Verification items for the finished model (mm, model axes). Face numbers are marked on the shaded views. A direction names the side the tool comes from. Give positions to 0.01 mm unless a question says otherwise; leave off trailing zeros. Order: outer loops, then holes, each group sorted by start corner. A loop starts at its lowest first (then second) coordinate and runs counter-clockwise, first axis right, second up. Notation, with made-up numbers: (62.25, 75.25) - (118.25, 75.25) arc R26 ccw to (118.25, 108.25) - close; hole circle Ø7 at (24, -5.5). An arc over 180 degrees is marked (long way). Answer as a JSON object with one key per item and string values.
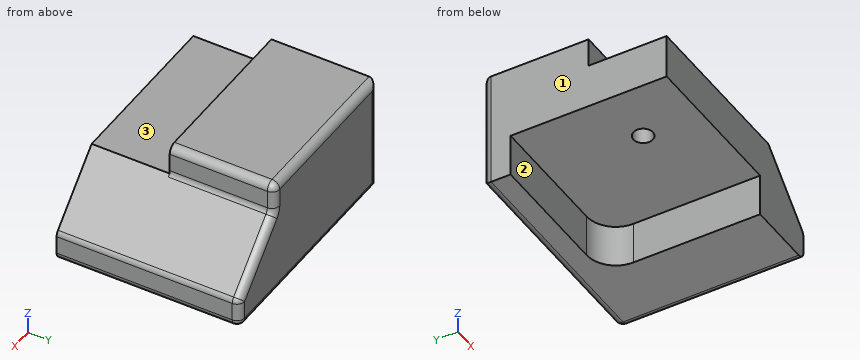
```python
from build123d import *

# Parameters (mm, degrees)
SKETCH2_W           = 14.859
SKETCH2_H           = 11.938
BOSS_EXTRUDE1_DEPTH = 7.62
CUT_EXTRUDE2_DEPTH  = 2.794
CUT_EXTRUDE3_DEPTH  = 1.905
CUT_EXTRUDE4_DEPTH  = 12.938
FILLET1_R           = 0.508
SKETCH7_R           = 0.635
CUT_EXTRUDE13_DEPTH = 1.905


with BuildPart() as part:
    # Sketch2 → Boss-Extrude1 (new body)
    with BuildSketch(Plane.XY):
        with Locations((7.4295, 5.969)):
            Rectangle(SKETCH2_W, SKETCH2_H)
    extrude(amount=BOSS_EXTRUDE1_DEPTH)

    # Sketch4 → Cut-Extrude2 (cut)
    with BuildSketch(Plane(origin=(0, 0, 0), x_dir=(-1, 0, 0), z_dir=(0, 0, -1))):
        with BuildLine():
            Line((0, 0), (-10.16, 0))
            Line((-10.16, 0), (-10.16, 8.255))
            ThreePointArc((-10.16, 8.255), (-9.602038418, 9.602038418), (-8.255, 10.16))
            Line((-8.255, 10.16), (0, 10.16))
            Line((0, 10.16), (0, 0))
        make_face()
    extrude(amount=-CUT_EXTRUDE2_DEPTH, mode=Mode.SUBTRACT)

    # Sketch5 → Cut-Extrude3 (cut)
    with BuildSketch(Plane.XY.offset(7.62)):
        Polygon((14.859, 11.938), (11.049, 11.938), (11.049, 5.08), (0, 5.08), (0, 0), (14.859, 0), align=None)
    extrude(amount=-CUT_EXTRUDE3_DEPTH, mode=Mode.SUBTRACT)

    # Sketch6 → Cut-Extrude4 (cut, through all)
    with BuildSketch(Plane(origin=(0, 11.938, 0), x_dir=(1, 0, 0), z_dir=(0, 1, 0))):
        Polygon((14.859, -1.905), (11.049, -5.715), (14.859, -5.715), align=None)
    extrude(amount=-CUT_EXTRUDE4_DEPTH, mode=Mode.SUBTRACT)

    # Fillet1
    fillet1_edges = [part.edges().sort_by_distance(p)[0] for p in [
        (5.5245, 11.938, 7.62),
        (11.049, 11.938, 6.6675),
        (11.049, 8.509, 5.715),
        (11.049, 8.509, 7.62),
        (7.4295, 11.938, 0),
        (14.859, 11.938, 0.9525),
        (14.859, 5.969, 0),
        (12.954, 11.938, 3.81),
        (14.859, 5.969, 1.905),
        (0, 11.938, 3.81),
    ]]
    fillet(fillet1_edges, radius=FILLET1_R)

    # Sketch7 → Cut-Extrude13 (cut)
    with BuildSketch(Plane(origin=(0, 0, 2.794), x_dir=(-1, 0, 0), z_dir=(0, 0, -1))):
        with Locations((-3.81, 3.81)):
            Circle(SKETCH7_R)
    extrude(amount=-CUT_EXTRUDE13_DEPTH, mode=Mode.SUBTRACT)


solid = part.part
```
(1) Access from +Z, -Z, +X, -X, +Y, -Y to the whole of each face (thin tool, end or side, straight path). Record for the marked faces 1, 2 and 3.
Computed values:
{"face 1": "+Z, -Z, -X, +Y, -Y", "face 2": "-Z, -X, -Y", "face 3": "+Z, +X, -X, -Y"}
(2) Section check D-D (y = 0.5). Record the cut outline in (x, z) (3 decimals), then the cut area to 3 significant figures.
Computed values:
{"outline": "(0, 2.794) - (10.16, 2.794) - (10.16, 0) - (14.351, 0) arc R0.508 ccw to (14.859, 0.508) - (14.859, 1.695) arc R0.508 ccw to (14.71, 2.054) - (11.049, 5.715) - (0, 5.715) - close", "area": "49.2 mm²"}
(3) Material ranges on line 1 along Y through (x, z) = (3.81, 3.95) (3 decimals); line 2 along Z through (x, y) = (4.75, 8); line 3 along Z through (x, y) = (3.75, 1) (3 decimals), recorded low to high. Write a range as [from, to].
Computed values:
{"line 1": "y = [0, 3.175], [4.445, 11.938]", "line 2": "z = [2.79, 7.62]", "line 3": "z = [2.794, 5.715]"}
(4) Gauge pin test, flat ends, axial feed: pin 1 Ø1 at (x, y) = (3.81, 3.81) entering from -Z; pin 2 Ø2.5 at (x, y) = (7, 2.5) entering from +Z (3 decimals); pin 3 Ø1.5 at (x, y) = (8, 6.5) entering from -Z. Record the tip position at first contact, or that the pin passes through.
Computed values:
{"pin 1": "stops at z = 4.7", "pin 2": "stops at z = 5.715", "pin 3": "stops at z = 2.79"}
(5) Section check A-A (y = 3.81). Record the cut outline in (x, z) (3 decimals).
Computed values:
{"outline": "(0, 2.794) - (3.175, 2.794) - (3.175, 4.699) - (4.445, 4.699) - (4.445, 2.794) - (10.16, 2.794) - (10.16, 0) - (14.351, 0) arc R0.508 ccw to (14.859, 0.508) - (14.859, 1.695) arc R0.508 ccw to (14.71, 2.054) - (11.049, 5.715) - (0, 5.715) - close"}
(6) Section check C-C (y = 6.75). Record the cut outline in (x, z).
Computed values:
{"outline": "(0, 2.79) - (10.16, 2.79) - (10.16, 0) - (14.35, 0) arc R0.51 ccw to (14.86, 0.51) - (14.86, 1.69) arc R0.51 ccw to (14.71, 2.05) - (11.2, 5.57) arc R0.51 cw to (11.05, 5.93) - (11.05, 7.11) arc R0.51 ccw to (10.54, 7.62) - (0, 7.62) - close"}
(7) Section check B-B (x = 2.5). Record the cut outline in (y, z) (3 decimals).
Computed values:
{"outline": "(0, 2.794) - (10.16, 2.794) - (10.16, 0) - (11.43, 0) arc R0.508 ccw to (11.938, 0.508) - (11.938, 7.112) arc R0.508 ccw to (11.43, 7.62) - (5.08, 7.62) - (5.08, 5.715) - (0, 5.715) - close"}
